Geometry: see drawing. Coordinates: mm, zero at the bounding-box minimum. A direction names the side the tool comes from. Round coordinates to 2 decimals unless told otherwise and drop trailing zeros. Order: outer loops, then holes, each group sorted by start corner. A loop starts at its lowest first (then second) coordinate and runs counter-clockwise, first axis right, second up. Notation, with made-up numbers: (-26.75, 52) - (-0.75, 52) arc R38 ccw to (-0.75, 91) - close; hole circle Ø4 at (-25, 42.5). An arc over 180 degrees is marked (long way). Put each result on its own line as item: value. Start each with the question number.
1) Access query for the marked faces 1 and 2. Directions: +Z, -Z, +X, -X, +Y, -Y. A direction counts if a zero-diameter tool reaches every point of the face in a straight line with its end or side. Return the directions, or none.
2) Section C-C on y = 26.5. Output: boundary loops of the cut face in (x, z), then the cut area to 3 significant figures.
3) Line query: probe 1 along X at (y, z) = (31, 5.5); probe 2 along Y at (x, z) = (3.5, 24); probe 3 along X at (y, z) = (12, 2.5). Output: solid intervals per line, ascending. Write a range as [from, to].
4) Section B-B on z = 20.5. Output: boundary loops of the cut face in (x, y), then the cut area to 3 significant figures.
5) Section D-D on x = 10.5. Output: boundary loops of the cut face in (y, z), then the cut area to 3 significant figures.
6) Section A-A on x = 22.5. Output: boundary loops of the cut face in (y, z), then the cut area to 3 significant figures.
7) Contact query for a flat-ended pin moving along its axis: P1, Ø8, axis at x = 13.5, z = 17.5, coming from the -Y side. Output: stop coordinate, or through.
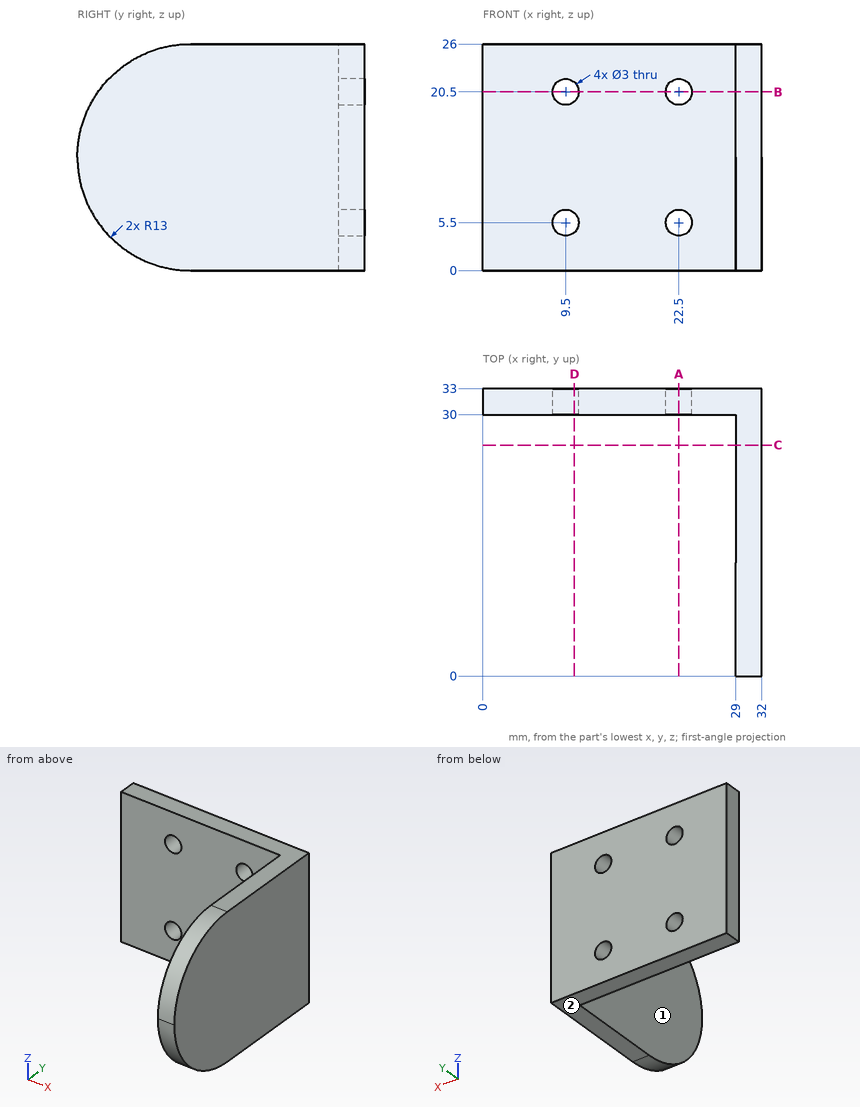
Answer sheet:
1. face 1: +Z, -Z, -X, -Y
1. face 2: -Z, +X, -X, +Y, -Y
2. outline: (29, 0) - (32, 0) - (32, 26) - (29, 26) - close
2. area: 78.0 mm^2
3. probe 1: [0, 8], [11, 21], [24, 32]
3. probe 2: [30, 33]
3. probe 3: [29, 32]
4. outline: (0, 30) - (8, 30) - (8, 33) - (0, 33) - close; (11, 30) - (21, 30) - (21, 33) - (11, 33) - close; (24, 30) - (29, 30) - (29, 2.38) - (32, 2.38) - (32, 33) - (24, 33) - close
4. area: 161 mm^2
5. outline: (30, 0) - (33, 0) - (33, 4.38) - (30, 4.38) - close; (30, 6.62) - (33, 6.62) - (33, 19.38) - (30, 19.38) - close; (30, 21.62) - (33, 21.62) - (33, 26) - (30, 26) - close
5. area: 64.6 mm^2
6. outline: (30, 0) - (33, 0) - (33, 4) - (30, 4) - close; (30, 7) - (33, 7) - (33, 19) - (30, 19) - close; (30, 22) - (33, 22) - (33, 26) - (30, 26) - close
6. area: 60.0 mm^2
7. P1: y = 30
